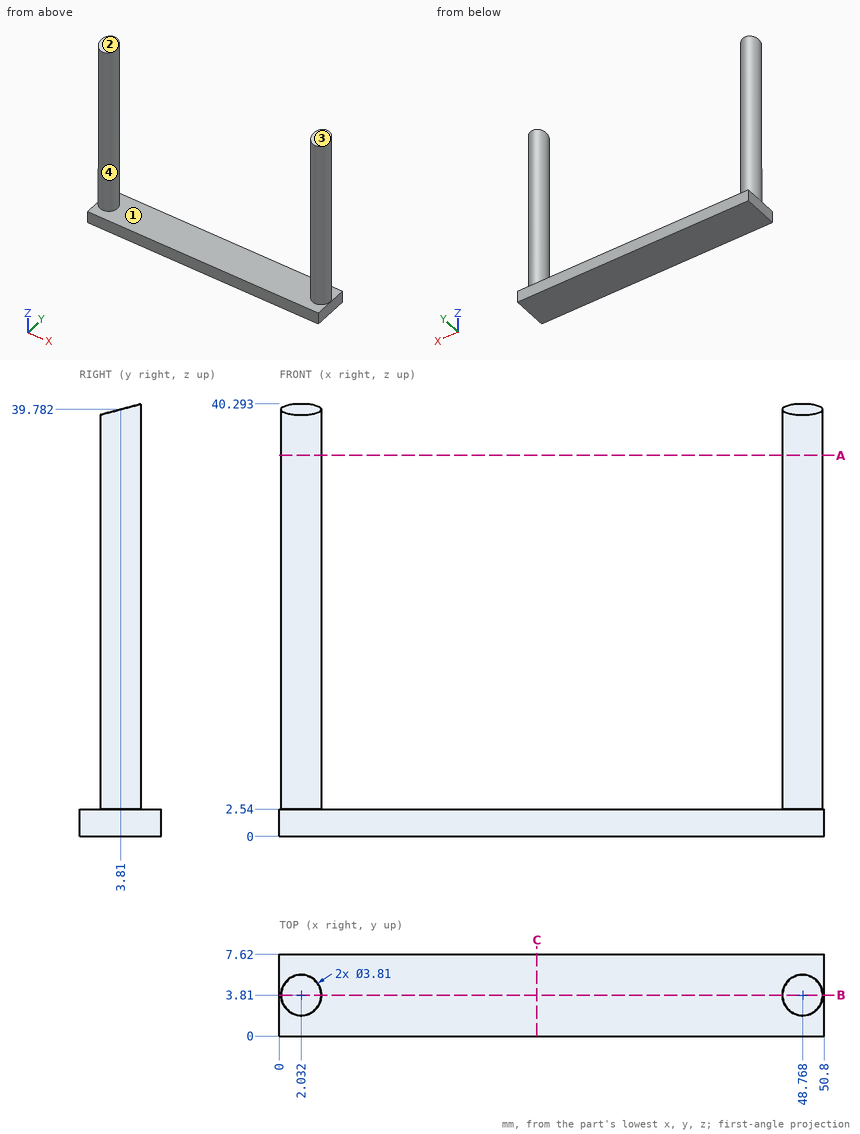
Job drawing, mm, ordinate dimensions from the low corner. One solid piece. A direction names the side the tool comes from. Give positions to 0.01 mm unless a question says otherwise; leave off trailing zeros. Loops run counter-clockwise (first coordinate to the right, second up) from the corner with the lowest first, then second, coordinate; pieces in that order, holes last. Notation, with made-up numbers: M -24,-10 L -4,-10 A24 ccw -4,26 Z; hole C 40.25,-22.5 d3. An arc over 180 degrees is marked long. Put each result on its own line as item: value. Start each with the question number.
1) Saw through at C-C (x = 24). List the corners of the cut face in (y, z).
2) Flat gauge pins, fed straight in: pin 1 (3 mm diameter, centred on y = 3.5, z = 8.5, fed in from -X); pin 2 (1 mm diameter, centred on y = 2, z = 19.5, fed in from -X); pin 3 (1 mm diameter, centred on y = 2, z = 27, fed in from +X). Where does each tip first touch, or does it go through?
3) Probe probe 1 along Z at (x, y) = (40.5, 6.75); probe 2 along X at (y, z) = (5, 11) (1 decimal); probe 3 along X at (y, z) = (4, 6). List the from-to ranges inside material, lowest first.
4) Saw through at B-B (y = 3.81). List the corners of the cut face in (x, z), then the cut area to 3 significant figures.
5) 3-axis set-ups, long thin cutter, end or side, ignore diameter. For the marked faces 3 and 4: which of +Z, -Z, +X, -X, +Y, -Y reach the whole face in a straight line?
6) Saw through at A-A (z = 35.5). List the corners of the cut face in (x, y) (1 decimal), then the cut area to 3 significant figures.
7) Pull direction X, two halves, no side cores. Call the marked faces 1 and 2: +X half, -X half, draft (parallel to the pull), parting line (faces both ways), or undercut.
Numbers:
1. outline: M 0,0 L 7.62,0 L 7.62,2.54 L 0,2.54 Z
2. pin 1: x = 0.13
2. pin 2: x = 0.65
2. pin 3: x = 50.15
3. probe 1: 0 to 2.54
3. probe 2: 0.5 to 3.5, 47.3 to 50.3
3. probe 3: 0.14 to 3.93, 46.87 to 50.66
4. outline: M 0,0 L 50.8,0 L 50.8,2.54 L 50.67,2.54 L 50.67,39.78 L 46.86,39.78 L 46.86,2.54 L 3.94,2.54 L 3.94,39.78 L 0.13,39.78 L 0.13,2.54 L 0,2.54 Z
4. area: 413 mm^2
5. face 3: +Z, +X, -X, -Y
5. face 4: +Z
6. outline: C 2,3.8 d3.8; C 48.8,3.8 d3.8
6. area: 22.8 mm^2
7. face 1: undercut
7. face 2: draft
